Source: CAD feature listing. Evaluate the final solid. Frame: model axes, mm. Give positions to 0.01 mm unless a question says otherwise; leave off trailing zeros. Write each loop counter-clockwise with the first axis right and the second up, starting at its lowest first coordinate (ties: lowest second). Pieces come first, ordered by that corner, then holes. Notation, with made-up numbers: M 2.25,86 L 51.25,86 A30 ccw 51.25,115 Z; hole C -1,38 d9. An arc over 180 degrees is marked long. Answer as a JSON object with one key per item and string values. Group by question number.
```python
from build123d import *

# Parameters (mm, degrees)
SALIENTE_EXTRUIR1_DEPTH = 3
CROQUIS2_R              = 1.5
CORTAR_EXTRUIR1_DEPTH   = 4
CROQUIS3_W              = 40.415918572
CROQUIS3_H              = 97.617868818
CROQUIS3_W_2            = 62.592919448
CROQUIS3_H_2            = 252.082446821
CORTAR_EXTRUIR2_DEPTH   = 18


with BuildPart() as part:
    # Croquis1 → Saliente-Extruir1 (new body)
    with BuildSketch(Plane(origin=(0, 0, 0), x_dir=(1, 0, 0), z_dir=(0, 1, 0))):
        Polygon((31, -188.773821898), (-31, -188.773821898), (-16.554484331, 188.773821898), (16.554484331, 188.773821898), align=None)
    extrude(amount=SALIENTE_EXTRUIR1_DEPTH)

    # Croquis2 → Cortar-Extruir1 (cut)
    with BuildSketch(Plane(origin=(0, 3, 0), x_dir=(1, 0, 0), z_dir=(0, 1, 0))):
        with Locations(Location((0, 78.297657431, 0), (0, 0, 270))):
            Circle(CROQUIS2_R)
        with Locations(Location((-18, 78.297657431, 0), (0, 0, 270))):
            Circle(CROQUIS2_R)
        with Locations(Location((18, 78.297657431, 0), (0, 0, 270))):
            Circle(CROQUIS2_R)
    extrude(amount=-CORTAR_EXTRUIR1_DEPTH, mode=Mode.SUBTRACT)

    # Croquis3 → Cortar-Extruir2 (cut)
    with BuildSketch(Plane(origin=(0, 3, 0), x_dir=(1, 0, 0), z_dir=(0, 1, 0))):
        with Locations((0, 142.095624348)):
            Rectangle(CROQUIS3_W, CROQUIS3_H)
        with Locations((0.296459724, -62.732598488)):
            Rectangle(CROQUIS3_W_2, CROQUIS3_H_2)
    extrude(amount=-CORTAR_EXTRUIR2_DEPTH, mode=Mode.SUBTRACT)


solid = part.part
```
(1) Ray query, L1, parallel to X at y = 0.9, z = -78.75; L2, parallel to Z at x = -17.5, y = 1.35; L3, parallel to X at y = 1.85, z = -86.5. Return the intervals inside material, ascending. Write a range as [from, to].
(2) Section B-B, the plane y = 2.5. Return loops of the section in (x, z).
(3) Pull-direction query (Z, two-part tool) for faces 1 (the flat face through (0, 2, -63.309)), 2 (the flat face through (20.773, 1.479, -78.508)), 3 (the cylindrical face through (0.451, 1.521, -76.867)); classes: pulls with the +Z half, pulls with the -Z half, needs draft (parallel to the pull), parting line crosses it, or undercut.
(4) Section A-A, the plane x = 18. Return loops of the section in (y, z).
(5) Section C-C, the plane z = -77.5. Return loops of the section in (x, y).
(6) Section D-D, the plane z = -89.25. Return loops of the section in (x, y), plus the area to 3 significant figures.
(7) Contact query for flat-ended pins moving along their axis: pin 1 Ø1.5 at (y, z) = (1.5, -72.5) entering from -X; pin 2 Ø3.5 at (x, z) = (18, -78.3) entering from -Y. Output: stop coordinate, or through.
Reported:
{
 "1": {"L1": "x = [-20.76, -19.43], [-16.57, -1.43], [1.43, 16.57], [19.43, 20.76]", "L2": "z = [-93.29, -79.71], [-76.88, -63.31]", "L3": "x = [-20.47, 20.47]"},
 "2": {"outline": "M -21.35,-63.31 L -20.21,-93.29 L 20.21,-93.29 L 21.35,-63.31 Z; hole C -18,-78.3 d3; hole C 0,-78.3 d3; hole C 18,-78.3 d3"},
 "3": {"face 1": "pulls with the +Z half", "face 2": "pulls with the -Z half", "face 3": "undercut"},
 "4": {"outline": "M 0,-93.29 L 3,-93.29 L 3,-79.8 L 0,-79.8 Z; M 0,-76.8 L 3,-76.8 L 3,-63.31 L 0,-63.31 Z"},
 "5": {"outline": "M -20.81,0 L -19.27,0 L -19.27,3 L -20.81,3 Z; M -16.73,0 L -1.27,0 L -1.27,3 L -16.73,3 Z; M 1.27,0 L 16.73,0 L 16.73,3 L 1.27,3 Z; M 19.27,0 L 20.81,0 L 20.81,3 L 19.27,3 Z"},
 "6": {"outline": "M -20.36,0 L 20.36,0 L 20.36,3 L -20.36,3 Z", "area": "122 mm2"},
 "7": {"pin 1": "stops at x = -21.03", "pin 2": "stops at y = 0"}
}
